from build123d import *

# Parameters (mm, degrees)
SKETCH1_W             = 160
SKETCH1_H             = 110
BOSS_EXTRUDE1_DEPTH   = 0.508
M12_CLEARANCE_HOLE1_D = 14
CUT_EXTRUDE1_DEPTH    = 98.083768283
M20_CLEARANCE_HOLE1_D = 22


with BuildPart() as part:
    # Sketch1 → Boss-Extrude1 (new body)
    with BuildSketch(Plane(origin=(0, 0, 0), x_dir=(0, 0, -1), z_dir=(1, 0, 0))):
        Rectangle(SKETCH1_W, SKETCH1_H)
    extrude(amount=BOSS_EXTRUDE1_DEPTH)

    # M12 Clearance Hole1 (through all)
    with Locations(Plane(origin=(0.508, 0, 0), x_dir=(0, 0, -1), z_dir=(1, 0, 0))):
        with Locations((-66, 40), (66, 40), (66, -40), (-66, -40)):
            Hole(M12_CLEARANCE_HOLE1_D / 2)

    # Sketch4 → Cut-Extrude1 (cut, through all)
    with BuildSketch(Plane(origin=(0.508, 0, 0), x_dir=(0, 0, -1), z_dir=(1, 0, 0))):
        with BuildLine():
            Line((2, 28), (2, -28))
            ThreePointArc((2, -28), (-5, -35), (-12, -28))
            Line((-12, -28), (-12, 28))
            ThreePointArc((-12, 28), (-5, 35), (2, 28))
        make_face()
    extrude(amount=-CUT_EXTRUDE1_DEPTH, mode=Mode.SUBTRACT)

    # M20 Clearance Hole1 (through all)
    with Locations(Plane(origin=(0.508, 0, 0), x_dir=(0, 0, -1), z_dir=(1, 0, 0))):
        with Locations((64, 12), (64, -12)):
            Hole(M20_CLEARANCE_HOLE1_D / 2)


solid = part.part
Model file for the job. Use its own axes, mm. A direction names the side the tool comes from. Give positions to 0.01 mm unless a question says otherwise; leave off trailing zeros. Order: outer loops, then holes, each group sorted by start corner. A loop starts at its lowest first (then second) coordinate and runs counter-clockwise, first axis right, second up. Notation, with made-up numbers: (29, -16) - (34, -16) arc R18 cw to (34, -5) - close; hole circle Ø8 at (74, 78). An arc over 180 degrees is marked (long way). One line per item, written item: value.
Item 1: Wall check: line 1 (Y direction, x = 0.35, z = 66); line 2 (Z direction, x = 0.2, y = 17.5); line 3 (Y direction, x = 0.45, z = -64). Give the ranges that are in metal, low to high.
Response values:
line 1: -55 to -47, -33 to 33, 47 to 55
line 2: -80 to -73.53, -54.47 to -2, 12 to 80
line 3: -55 to -46.71, -33.29 to -23, -1 to 1, 23 to 33.29, 46.71 to 55
Item 2: Slice it at A-A (y = 40). List the corners of the cut face in (x, z), then the cut area to 3 significant figures.
Response values:
outline: (0, -80) - (0.51, -80) - (0.51, -73) - (0, -73) - close; (0, -59) - (0.51, -59) - (0.51, 59) - (0, 59) - close; (0, 73) - (0.51, 73) - (0.51, 80) - (0, 80) - close
area: 67.1 mm2
Item 3: Tool access for faces 4 (the cylindrical face through (0.26, -35, 4.85)), 5 (the flat face through (0.508, 1, 19)): list every direction of +Z, -Z, +X, -X, +Y, -Y with a clear straight run to the whole face (end or side of a thin tool).
Response values:
face 4: +X, -X
face 5: +Z, -Z, +X, +Y, -Y
Item 4: Slice it at B-B (z = 5). List the corners of the cut face in (x, y), then the cut area to 3 significant figures.
Response values:
outline: (0, -55) - (0.51, -55) - (0.51, -35) - (0, -35) - close; (0, 35) - (0.51, 35) - (0.51, 55) - (0, 55) - close
area: 20.3 mm2
Item 5: Pin check, flat tip, straight feed: pin 1 Ø11 at (y, z) = (40, -66) entering from -X. Stop position of the tip, or through.
Response values:
pin 1: through
Item 6: Slice it at C-C (x = 0.25). List the corners of the cut face in (y, z), then the cut area to 3 significant figures.
Response values:
outline: (-55, -80) - (55, -80) - (55, 80) - (-55, 80) - close; hole circle Ø14 at (-40, -66); hole circle Ø14 at (-40, 66); hole (-28, -2) - (28, -2) arc R7 ccw to (28, 12) - (-28, 12) arc R7 ccw to start; hole circle Ø22 at (-12, -64); hole circle Ø22 at (12, -64); hole circle Ø14 at (40, -66); hole circle Ø14 at (40, 66)
area: 15,300 mm2
Item 7: Two-plate mould, pull along Z, no slides. Class faces 1 (the flat face through (0, 1, 19)), 2 (the cylindrical face through (0.25, 5.31, -72.73)), 3 (the cylindrical face through (0.26, 35, 5.15)): released by +Z, released by -Z, zero draft, split by the parting line, or undercut.
Response values:
face 1: zero draft
face 2: undercut
face 3: undercut
Item 8: Slice it at D-D (z = 66). List the corners of the cut face in (x, y).
Response values:
outline: (0, -55) - (0.51, -55) - (0.51, -47) - (0, -47) - close; (0, -33) - (0.51, -33) - (0.51, 33) - (0, 33) - close; (0, 47) - (0.51, 47) - (0.51, 55) - (0, 55) - close
